Autodesk Inventor part; units mm, degrees
ref_plane "YZ Plane" through (0, 0, 0) normal (1, 0, 0) x (0, 1, 0)
ref_plane "XZ Plane" through (0, 0, 0) normal (0, 1, 0) x (-1, 0, 0)
ref_plane "XY Plane" through (0, 0, 0) normal (0, 0, 1) x (1, 0, 0)
sketch "Sketch1" plane through (0, 0, 0) normal (1, 0, 0) x (0, 1, 0)
  circle A0 centre (0, 0) radius 10
  circle A1 centre (0, 0) radius 12
  circle A2 centre (0, 5) radius 1.5
  circle A3 centre (0, -5) radius 1.5
  line L0 (0, 5) -> (0, -5) construction
  dimension "d0" = 20
  dimension "d1" = 2
  dimension "d2" = 3
  dimension "d3" = 10
extrude "Extrusion1" add sketch "Sketch1" along normal blind 3.5 contours A0 | A1
extrude "Extrusion2" add sketch "Sketch1" against normal blind 6 contours A1
sketch "Sketch2" plane through (3.5, 0, 0) normal (1, 0, 0) x (0, 0, -1)
  circle A0 centre (0, 0) radius 12
  circle A1 centre (-5, 0) radius 1.5
  circle A2 centre (5, 0) radius 1.5
  circle A3 centre (0, 11.8) radius 3.9
  circle A4 centre (0, 0) radius 12
  line L0 (-10.2593, 6.2247) -> (-8.5634, 9.0198)
  line L1 (-7.6474, 10.1301) -> (-2.6198, 14.6891)
  arc A5 (-7.6474, 10.1301) -> (-8.5634, 9.0198) centre (-4.2887, 6.4262) ccw
  line L2 (0, 0) -> (0, 4.7438)
  line L3 (10.2593, 6.2247) -> (8.5634, 9.0198)
  line L4 (7.6474, 10.1301) -> (2.6198, 14.6891)
  arc A6 (8.5634, 9.0198) -> (7.6474, 10.1301) centre (4.2887, 6.4262) ccw
  point P0 (0.4335, 15.6758)
  point P1 (10.2649, 6.2155)
  point P2 (-10.2593, 6.2247)
  point P3 (10.2593, 6.2247)
  point P4 (-3.8748, 11.3572)
  point P5 (3.8748, 11.3572)
  dimension "d10" = 5
  dimension "d11" = 11.8
  dimension "d12" = 7.8
extrude "Extrusion3" add sketch "Sketch2" along normal blind 7
properties part number "CIRCULAR_FIN_DE_CARRERA" material "Steel, Mild, Welded"
Source: CAD feature listing. Evaluate the final solid. Frame: model axes, mm. A direction names the side the tool comes from. Round coordinates to 2 decimals unless told otherwise and drop trailing zeros. Order: outer loops, then holes, each group sorted by start corner. A loop starts at its lowest first (then second) coordinate and runs counter-clockwise, first axis right, second up. Notation, with made-up numbers: (-22.5, 64) -> (-6.5, 64) arc R15 cw to (-6.5, 82) -> close; hole circle Ø4 at (77.25, 71). An arc over 180 degrees is marked (long way). Answer as CSV lines item,"result".
Item 1: Pull-direction query (Y, two-part tool) for faces 1 (the face through (6.951, 7.603, 9.423)), 2 (the face through (0, 0, 0)), 3 (the face through (10.5, 2, 0)); classes: pulls with the +Y half, pulls with the -Y half, needs draft (parallel to the pull), parting line crosses it, or undercut.
A:
face 1,"pulls with the +Y half"
face 2,"undercut"
face 3,"needs draft"
Item 2: Section B-B, the plane x = 4. Return loops of the section in (y, z).
A:
outline,"(6.22, -10.26) -> (9.02, -8.56) arc R5 ccw to (10.13, -7.65) -> (14.69, -2.62) arc R3.9 ccw to (14.69, 2.62) -> (10.13, 7.65) arc R5 ccw to (9.02, 8.56) -> (6.22, 10.26) arc R12 ccw (long way) to start; hole circle Ø3 at (0, -5); hole circle Ø3 at (0, 5)"
Item 3: Pin query (flat end, axial travel): pin 1 Ø3 at (x, y) = (0, 11.5) entering from +Z; pin 2 Ø5 at (x, z) = (-2, -4) entering from +Y; pin 3 Ø10.5 at (y, z) = (9, -4) entering from -X; pin 4 Ø6 at (x, z) = (-1.5, 7.5) entering from -Y. Return the tip coordinate at first contact, or that it passes through.
A:
pin 1,"z = 6.63"
pin 2,"y = 11.91"
pin 3,"x = -6"
pin 4,"y = -11.12"
Item 4: Section D-D, the plane y = 3.25. Return loops of the section in (x, z).
A:
outline,"(-6, -11.55) -> (10.5, -11.55) -> (10.5, 11.55) -> (-6, 11.55) -> (-6, 9.46) -> (0, 9.46) -> (0, -9.46) -> (-6, -9.46) -> close"
Item 5: Reachability of faces 4 (the face through (7, 15.7, 0)), 5 (the face through (-2.96, -2.17, -9.76)), 6 (the face through (3.5, 13, 0)) from +Z, -Z, +X, -X, +Y, -Y: full face, straight path, thin tool, end or side. Return the list, or none.
A:
face 4,"+X, -X, +Y"
face 5,"-X"
face 6,"-X, +Y"
Item 6: Section C-C, the plane z = -5. Return loops of the section in (x, y).
A:
outline,"(-6, -10.91) -> (10.5, -10.91) -> (10.5, -1.5) -> (0, -1.5) -> (0, -8.66) -> (-6, -8.66) -> close; (-6, 8.66) -> (0, 8.66) -> (0, 1.5) -> (10.5, 1.5) -> (10.5, 12.53) -> (3.5, 12.53) -> (3.5, 10.91) -> (-6, 10.91) -> close"
Item 7: Line query: L1, parallel to Z at x = 1.7, y = 0; L2, parallel to Z at x = -4.6, y = 0; L3, parallel to Z at x = 8, y = 0.5. Output: solid intervals per line, ascending.
A:
L1,"-12 to -6.5, -3.5 to 3.5, 6.5 to 12"
L2,"-12 to -10, 10 to 12"
L3,"-11.99 to -6.41, -3.59 to 3.59, 6.41 to 11.99"
Item 8: Section A-A, the plane z = 0. Return loops of the section in (x, y), plus the area to 3 significant figures.
A:
outline,"(-6, -12) -> (10.5, -12) -> (10.5, 15.7) -> (3.5, 15.7) -> (3.5, 12) -> (-6, 12) -> (-6, 10) -> (0, 10) -> (0, -10) -> (-6, -10) -> close"
area,"302 mm²"
